Geometry: final body of the model. Coordinates: model frame, mm. Face numbers are marked on the shaded views. A direction names the side the tool comes from. Coordinates: 2 decimals unless noted, no trailing zeros. Loops run counter-clockwise (first coordinate to the right, second up) from the corner with the lowest first, then second, coordinate; pieces in that order, holes last. Notation, with made-up numbers: (16.25, 1) - (52.25, 1) arc R28 cw to (52.25, 24) - close; hole circle Ø10 at (-14.75, 37). An arc over 180 degrees is marked (long way). Return JSON: item names as keys, results as strings.
from build123d import *

# Parameters (mm, degrees)
SKETCH_1_R          = 2.5
EXTRUDE_1_DEPTH     = 1.6
SKETCH_2_R          = 1.5
EXTRUDE_2_DEPTH     = 5
CUT_EXTRUDE_1_DEPTH = 1


with BuildPart() as part:
    # 草图1 → 凸台-拉伸1 (new body)
    with BuildSketch(Plane(origin=(0, 0, 0), x_dir=(1, 0, 0), z_dir=(0, 1, 0))):
        Circle(SKETCH_1_R)
    extrude(amount=EXTRUDE_1_DEPTH)

    # 草图2 → 凸台-拉伸2 (add)
    with BuildSketch(Plane(origin=(0, 1.6, 0), x_dir=(1, 0, 0), z_dir=(0, 1, 0))):
        Circle(SKETCH_2_R)
    extrude(amount=EXTRUDE_2_DEPTH)

    # 草图3 → 切除-拉伸1 (cut)
    with BuildSketch(Plane.XZ):
        with BuildLine():
            Line((-0.5, 1), (-0.5, 1.75))
            Line((-0.5, 1.75), (0.5, 1.75))
            Line((0.5, 1.75), (0.5, 1))
            ThreePointArc((0.5, 1), (0.646446609, 0.646446609), (1, 0.5))
            Line((1, 0.5), (1.75, 0.5))
            Line((1.75, 0.5), (1.75, -0.5))
            Line((1.75, -0.5), (1, -0.5))
            ThreePointArc((1, -0.5), (0.646446609, -0.646446609), (0.5, -1))
            Line((0.5, -1), (0.5, -1.75))
            Line((0.5, -1.75), (-0.5, -1.75))
            Line((-0.5, -1.75), (-0.5, -1))
            ThreePointArc((-0.5, -1), (-0.646446609, -0.646446609), (-1, -0.5))
            Line((-1, -0.5), (-1.75, -0.5))
            Line((-1.75, -0.5), (-1.75, 0.5))
            Line((-1.75, 0.5), (-1, 0.5))
            ThreePointArc((-1, 0.5), (-0.646446609, 0.646446609), (-0.5, 1))
        make_face()
    extrude(amount=-CUT_EXTRUDE_1_DEPTH, mode=Mode.SUBTRACT)


solid = part.part
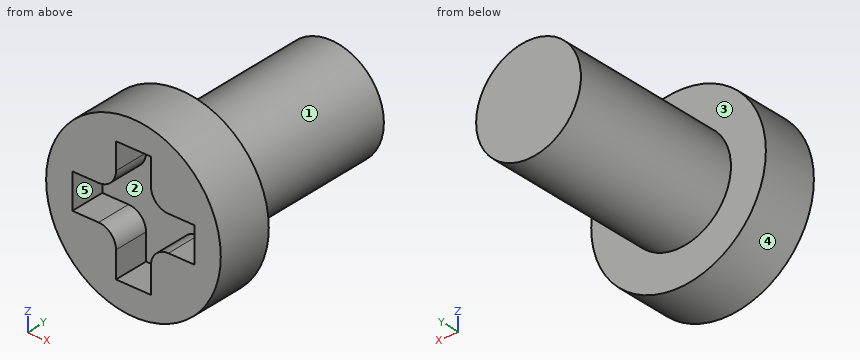
Item 1: Mould query, pull axis Z, two halves, no side actions, for the marked faces 1, 2 and 3. Classes: +Z half, -Z half, draft (parallel to the pull), parting line (faces both ways), or undercut.
Worked out:
{"face 1": "parting line", "face 2": "undercut", "face 3": "draft"}
Item 2: Section query B-B, the plane z = 0. Return loops of the section in (x, y), and give its area (3 significant figures).
Worked out:
{"outline": "(-2.5, 0) - (-1.75, 0) - (-1.75, 1) - (1.75, 1) - (1.75, 0) - (2.5, 0) - (2.5, 1.6) - (1.5, 1.6) - (1.5, 6.6) - (-1.5, 6.6) - (-1.5, 1.6) - (-2.5, 1.6) - close", "area": "19.5 mm^2"}
Item 3: First-contact query: pin 1 Ø1.5 at (y, z) = (5, 0.5) entering from +X; pin 2 Ø0.6 at (x, y) = (-1.5, 0.5) entering from -Z; pin 3 Ø0.6 at (x, y) = (1.5, 0.5) entering from +Z. Flat tips, straight axial feed; report the tip coordinate or a pass-through.
Worked out:
{"pin 1": "x = 1.5", "pin 2": "z = -2.19", "pin 3": "z = 2.19"}
Item 4: Section query D-D, the plane z = -1.95. Return loops of the section in (x, y).
Worked out:
{"outline": "(-1.56, 0) - (1.56, 0) - (1.56, 1.6) - (-1.56, 1.6) - close"}
Item 5: Reachability of the marked faces 4 and 5 from +Z, -Z, +X, -X, +Y, -Y: full face, straight path, thin tool, end or side. Return the list, or none.
Worked out:
{"face 4": "+Y, -Y", "face 5": "-Y"}
Item 6: Section query A-A, the plane x = 0. Return loops of the section in (y, z), and give its area (3 significant figures).
Worked out:
{"outline": "(0, -2.5) - (1.6, -2.5) - (1.6, -1.5) - (6.6, -1.5) - (6.6, 1.5) - (1.6, 1.5) - (1.6, 2.5) - (0, 2.5) - (0, 1.75) - (1, 1.75) - (1, -1.75) - (0, -1.75) - close", "area": "19.5 mm^2"}
Item 7: Ray query, probe 1 along Z at (x, y) = (-0.05, 3.25); probe 2 along Y at (x, z) = (-1.1, -1.8); probe 3 along X at (y, z) = (0.5, -0.4). Return the intervals inside material, ascending. Write a range as from..to.
Worked out:
{"probe 1": "-1.5..1.5", "probe 2": "0..1.6", "probe 3": "-2.47..-1.75, 1.75..2.47"}
Item 8: Section query C-C, the plane y = 2.5. Return loops of the section in (x, z).
Worked out:
{"outline": "circle Ø3 at (0, 0)"}
